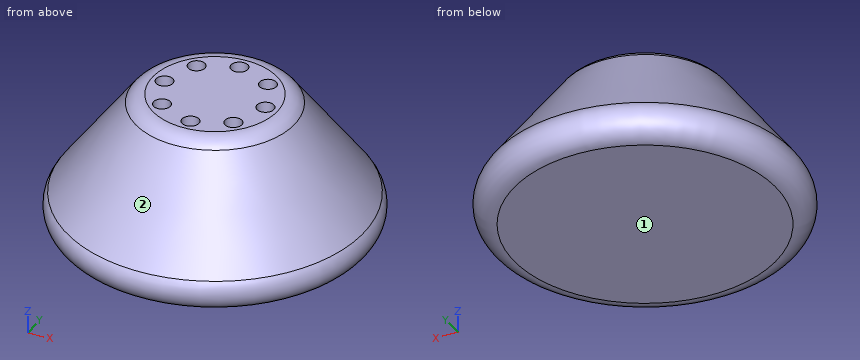
```python
from build123d import *

# Parameters (mm, degrees)
F2_R            = 5.08
F3_R            = 2.006915686
F4_DEPTH        = 25.4
F4_COPIES_COUNT = 8


# Not quite as in the source:
# - a pattern or mirror of a feature is missing from the dataset's text; its kind, count and spacing are read off the source's solid


with BuildPart() as f1:
    # F0 (on Front) → F1 (revolve)
    with BuildSketch(Plane.XZ):
        Polygon((0, 23.1683626771), (0, 55.6904152036), (-17.4122489989, 55.6904152036), (-41.3001254201, 23.1683626771), align=None)
    revolve(axis=Axis((0, 0, 39.4293889403), (0, 0, 1)))

    # F2
    f2_edges = [f1.edges().sort_by_distance(p)[0] for p in [
        (41.300125, 0, 23.168363),
        (17.412249, 0, 55.690415),
    ]]
    fillet(f2_edges, radius=F2_R)

    # F3 (on face) → F4 (cut)
    with BuildSketch(Plane.XY.offset(55.6904152036)):
        with Locations((-8.7765334174, 7.9615563154)):
            Circle(F3_R)
    f4 = extrude(amount=-F4_DEPTH, mode=Mode.SUBTRACT)

    # F4_copies: F4 ×8 about axis
    f4_copies_axis = Axis((0, 0, 0), (0, 0, 1))
    for i in range(1, F4_COPIES_COUNT):
        add(f4.rotate(f4_copies_axis, i * 360 / F4_COPIES_COUNT), mode=Mode.SUBTRACT)


solid = f1.part
```
Geometry: final body of the model. Coordinates: model frame, mm. Face numbers are marked on the shaded views. Give positions to 0.01 mm unless a question says otherwise; leave off trailing zeros. Use CSV: the item, a comma, the result in double quotes.
(1) Ray query, line 1 along X through (y, z) = (1, 37.5); line 2 along X through (y, z) = (-7, 43); line 3 along Y through (x, z) = (-1.5, 32.5). Return the intervals inside material, ascending. Write a range as [from, to].
From the geometry:
line 1,"[-30.76, -13.08], [-10.59, 9.87], [13.8, 30.76]"
line 2,"[-25.8, -8.9], [-7.03, 7.01], [10.54, 25.8]"
line 3,"[-34.41, 10.05], [13.62, 34.41]"
(2) First-contact query: P1, Ø1.5, axis at x = -26, y = -14, coming from the +Z side; P2, Ø2, axis at x = -3, z = 29, coming from the +Y side; P3, Ø3, axis at y = 0.5, z = 37, coming from the -X side. Flat tips, straight axial feed; report the tip coordinate or a pass-through.
From the geometry:
P1,"z = 40.21"
P2,"y = 36.28"
P3,"x = -32.24"
(3) Pull-direction query (Y, two-part tool) for the marked faces 1 and 2; classes: released by +Y, released by -Y, zero draft, split by the parting line, or undercut.
From the geometry:
face 1,"zero draft"
face 2,"split by the parting line"
(4) Cut plane A-A (z = 39.5). Count the separate pieces of the cut face and the enclosed holes in it, plus the area to 3 significant figures.
From the geometry:
separate pieces,"1"
enclosed holes,"8"
area,"2,600 mm^2"
